The model under review builds one solid part; all positions refer to its coordinate system, in mm. Face numbers are marked on the shaded views. A direction names the side the tool comes from. Round coordinates to 2 decimals unless told otherwise and drop trailing zeros. Order: outer loops, then holes, each group sorted by start corner. A loop starts at its lowest first (then second) coordinate and runs counter-clockwise, first axis right, second up. Notation, with made-up numbers: (67.5, -5.75) -> (110.5, -5.75) arc R19 ccw to (110.5, 27.25) -> close; hole circle Ø8 at (78.25, -11). An arc over 180 degrees is marked (long way). Return JSON: item names as keys, results as strings. Group by question number.
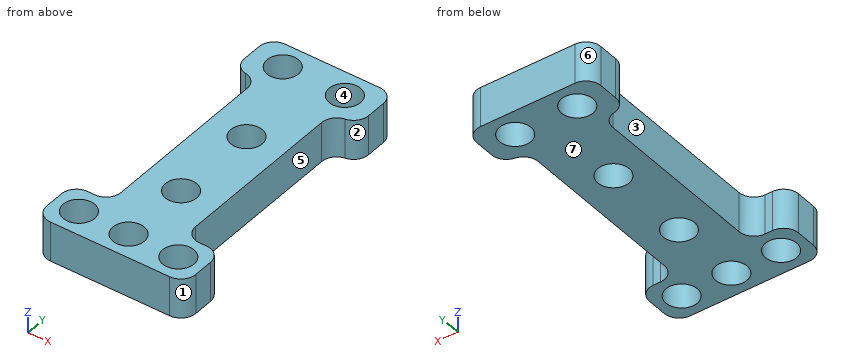
from build123d import *

# Parameters (mm, degrees)
F0_W      = 19.05
F0_H      = 63.5
F0_R      = 4.0132
F1_DEPTH  = 10.16
F2_R      = 4.0132
F3_DEPTH  = 25.4
F4_W      = 6.35
F4_H      = 12.7
F5_DEPTH  = 10.16
F7_DEPTH  = 25.4
F8_R      = 3.81
F9_R      = 3.81
F10_R     = 4.0132
F11_DEPTH = 25.4


with BuildPart() as f1:
    # F0 (on Top) → F1 (new body)
    with BuildSketch(Plane.XY):
        with Locations((0, 38.1)):
            Rectangle(F0_W, F0_H)
        Polygon((-19.05, -6.35), (19.05, -6.35), (19.05, 6.35), (9.525, 6.35), (-9.525, 6.35), (-19.05, 6.35), align=None)
        with Locations((-12.7, 0)):
            Circle(F0_R, mode=Mode.SUBTRACT)
        Circle(F0_R, mode=Mode.SUBTRACT)
        with Locations((12.7, 0)):
            Circle(F0_R, mode=Mode.SUBTRACT)
    extrude(amount=F1_DEPTH)

    # F2 (on face) → F3 (cut)
    with BuildSketch(Plane(origin=(0, 0, 0), x_dir=(1, 0, 0), z_dir=(0, 0, -1))):
        with Locations((0, -17.9832)):
            Circle(F2_R)
    extrude(amount=-F3_DEPTH, mode=Mode.SUBTRACT)

    # F4 (on face) → F5 (join)
    with BuildSketch(Plane(origin=(0, 0, 0), x_dir=(1, 0, 0), z_dir=(0, 0, -1))):
        with Locations((-12.7, -63.5)):
            Rectangle(F4_W, F4_H)
        with Locations((12.7, -63.5)):
            Rectangle(F4_W, F4_H)
    extrude(amount=-F5_DEPTH)

    # F6 (on face) → F7 (cut)
    with BuildSketch(Plane(origin=(0, 0, 0), x_dir=(1, 0, 0), z_dir=(0, 0, -1))):
        with BuildLine():
            ThreePointArc((-11.9507, -63.5), (-7.9375, -67.5132), (-3.9243, -63.5))
            Line((-3.9243, -63.5), (-11.9507, -63.5))
        make_face()
        with BuildLine():
            Line((-11.9507, -63.5), (-3.9243, -63.5))
            ThreePointArc((-3.9243, -63.5), (-7.9375, -59.4868), (-11.9507, -63.5))
        make_face()
        with BuildLine():
            Line((3.9243, -63.5), (11.9507, -63.5))
            ThreePointArc((11.9507, -63.5), (7.9375, -59.4868), (3.9243, -63.5))
        make_face()
        with BuildLine():
            ThreePointArc((3.9243, -63.5), (7.9375, -67.5132), (11.9507, -63.5))
            Line((11.9507, -63.5), (3.9243, -63.5))
        make_face()
    extrude(amount=-F7_DEPTH, mode=Mode.SUBTRACT)

    # F8
    f8_edges = [f1.edges().sort_by_distance(p)[0] for p in [
        (19.05, -6.35, 5.08),
        (-19.05, -6.35, 5.08),
        (-19.05, 6.35, 5.08),
        (19.05, 6.35, 5.08),
        (15.875, 57.15, 5.08),
        (15.875, 69.85, 5.08),
        (-15.875, 69.85, 5.08),
        (-15.875, 57.15, 5.08),
    ]]
    fillet(f8_edges, radius=F8_R)

    # F9
    f9_edges = [f1.edges().sort_by_distance(p)[0] for p in [
        (-9.525, 6.35, 5.08),
        (-9.525, 57.15, 5.08),
        (9.525, 6.35, 5.08),
        (9.525, 57.15, 5.08),
    ]]
    fillet(f9_edges, radius=F9_R)

    # F10 (on face) → F11 (cut)
    with BuildSketch(Plane(origin=(0, 0, 0), x_dir=(1, 0, 0), z_dir=(0, 0, -1))):
        with Locations((0, -40.4368)):
            Circle(F10_R)
    extrude(amount=-F11_DEPTH, mode=Mode.SUBTRACT)


solid = f1.part
Item 1: The part is to be moulded in two halves that separate along Y. For the marked faces 4, 5, 6 and 7, say which applies: +Y half, -Y half, draft (parallel to the pull), parting line (faces both ways), or undercut.
Item 2: Insertion check: pin 1 Ø6 at (y, z) = (11, 3) entering from +X; pin 2 Ø5 at (x, y) = (12.7, 0) entering from -Z; pin 3 Ø1 at (x, z) = (14, 5.5) entering from +Y; pin 4 Ø3 at (y, z) = (21.5, 3.5) entering from -X (3 decimals). Each pin has a flat end and moves straight along its axis. Give the tip position at first contact, or say it passes through.
Item 3: Consider section D-D on y = 63.5. State the section outline as (x, z) points (3 decimals), plus the area to 3 significant figures.
Item 4: Consider section A-A on x = 0. State the section outline as (y, z) points.
Item 5: Consider section B-B on y = 0. State the section outline as (x, z) points.
Item 6: For the marked faces 1, 2 and 3, list the 3-axis set-ups (+Z, -Z, +X, -X, +Y, -Y) from which the entire face can be reached by the end or side of a thin tool; tool diameter is ignored.
Item 7: Wall thickness on line 1 along Y through (x, z) = (0, 9); line 2 along Y through (x, z) = (-10.5, 4.75); line 3 along Y through (x, z) = (-15.5, 0.5): over which ranges is each line inside the solid? List them lowest first.
Item 8: Consider section C-C on x = 14.5. State the section outline as (y, z) points.
Values:
{
 "1": {"face 4": "undercut", "face 5": "undercut", "face 6": "+Y half", "face 7": "draft"},
 "2": {"pin 1": "x = 10.2", "pin 2": "through", "pin 3": "y = 69.57", "pin 4": "x = -9.525"},
 "3": {"outline": "(-15.875, 0) -> (-11.951, 0) -> (-11.951, 10.16) -> (-15.875, 10.16) -> close; (-3.924, 0) -> (3.924, 0) -> (3.924, 10.16) -> (-3.924, 10.16) -> close; (11.951, 0) -> (15.875, 0) -> (15.875, 10.16) -> (11.951, 10.16) -> close", "area": "159 mm^2"},
 "4": {"outline": "(-6.35, 0) -> (-4.01, 0) -> (-4.01, 10.16) -> (-6.35, 10.16) -> close; (4.01, 0) -> (13.97, 0) -> (13.97, 10.16) -> (4.01, 10.16) -> close; (22, 0) -> (36.42, 0) -> (36.42, 10.16) -> (22, 10.16) -> close; (44.45, 0) -> (69.85, 0) -> (69.85, 10.16) -> (44.45, 10.16) -> close"},
 "5": {"outline": "(-19.05, 0) -> (-16.71, 0) -> (-16.71, 10.16) -> (-19.05, 10.16) -> close; (-8.69, 0) -> (-4.01, 0) -> (-4.01, 10.16) -> (-8.69, 10.16) -> close; (4.01, 0) -> (8.69, 0) -> (8.69, 10.16) -> (4.01, 10.16) -> close; (16.71, 0) -> (19.05, 0) -> (19.05, 10.16) -> (16.71, 10.16) -> close"},
 "6": {"face 1": "+Z, -Z, +X, -Y", "face 2": "+Z, -Z, +X", "face 3": "+Z, -Z, -X"},
 "7": {"line 1": "-6.35 to -4.01, 4.01 to 13.97, 22 to 36.42, 44.45 to 69.85", "line 2": "-6.35 to -3.36, 3.36 to 7.61, 55.99 to 60.41, 66.59 to 69.85", "line 3": "-6.34 to -2.88, 2.88 to 6.34, 59.31 to 67.69"},
 "8": {"outline": "(-6.35, 0) -> (-3.59, 0) -> (-3.59, 10.16) -> (-6.35, 10.16) -> close; (3.59, 0) -> (6.35, 0) -> (6.35, 10.16) -> (3.59, 10.16) -> close; (58.03, 0) -> (68.97, 0) -> (68.97, 10.16) -> (58.03, 10.16) -> close"}
}
